```python
from build123d import *

# Parameters (mm, degrees)
SZKIC1_R                    = 23.5
DODANIE_WYCI_GNI_CIE1_DEPTH = 302
SZKIC2_R                    = 17.5
DODANIE_WYCI_GNI_CIE2_DEPTH = 50
SZKIC4_R                    = 17.5
DODANIE_WYCI_GNI_CIE3_DEPTH = 50
SZKIC5_R                    = 5.05
WYTNIJ_WYCI_GNI_CIE1_DEPTH  = 50
SFAZOWANIE1_SIZE            = 2
SZKIC8_R                    = 24
DODANIE_WYCI_GNI_CIE4_DEPTH = 42.129872
SZKIC12_R                   = 7
DODANIE_WYCI_GNI_CIE5_DEPTH = 61.69017
SZKIC6_R                    = 19
WYTNIJ_WYCI_GNI_CIE2_DEPTH  = 302
DODANIE_WYCI_GNI_CIE6_START = -50
SZKIC13_R                   = 7
DODANIE_WYCI_GNI_CIE6_DEPTH = 50


with BuildPart() as part:
    # Szkic1 → Dodanie-wyciągnięcie1 (new body)
    with BuildSketch(Plane(origin=(0, 0, 0), x_dir=(0, 0, -1), z_dir=(1, 0, 0))):
        Circle(SZKIC1_R)
    extrude(amount=DODANIE_WYCI_GNI_CIE1_DEPTH)

    # Szkic2 → Dodanie-wyciągnięcie2 (add)
    with BuildSketch(Plane.XY):
        with Locations(Location((31.5, -38, 0), (0, 0, 124.04773237))):
            Circle(SZKIC2_R)
    extrude(amount=DODANIE_WYCI_GNI_CIE2_DEPTH)

    # Szkic4 → Dodanie-wyciągnięcie3 (add)
    with BuildSketch(Plane(origin=(0, 0, 0), x_dir=(-1, 0, 0), z_dir=(0, 0, -1))):
        with Locations((-271.5, -38)):
            Circle(SZKIC4_R)
    extrude(amount=-DODANIE_WYCI_GNI_CIE3_DEPTH)

    # Szkic5 → Wytnij-wyciągnięcie1 (cut)
    with BuildSketch(Plane.XY.offset(50)):
        with Locations((31.5, -38)):
            Circle(SZKIC5_R)
        with Locations((271.5, -38)):
            Circle(SZKIC5_R)
    extrude(amount=-WYTNIJ_WYCI_GNI_CIE1_DEPTH, mode=Mode.SUBTRACT)

    # Sfazowanie1
    sfazowanie1_edges = [part.edges().sort_by_distance(p)[0] for p in [
        (26.45, -38, 0),
        (26.45, -38, 50),
        (266.45, -38, 0),
        (266.45, -38, 50),
    ]]
    chamfer(sfazowanie1_edges, length=SFAZOWANIE1_SIZE)

    # Szkic8 → Dodanie-wyciągnięcie4 (add)
    with BuildSketch(Plane(origin=(64.694528313, 23.5, 42), x_dir=(0.9969173337331281, 0, 0.07845909572784458), z_dir=(-0.07845909572784458, 0, 0.9969173337331281))):
        with Locations((0, -13.25)):
            Circle(SZKIC8_R)
    extrude(amount=-DODANIE_WYCI_GNI_CIE4_DEPTH)

    # Szkic12 → Dodanie-wyciągnięcie5 (add)
    with BuildSketch(Plane(origin=(-2.886875267, 0, 36.681228189), x_dir=(0.9969173337331281, 0, 0.07845909572784461), z_dir=(-0.07845909572784461, 0, 0.9969173337331281))):
        with Locations((67.790378694, 10.25)):
            Circle(SZKIC12_R)
    extrude(amount=DODANIE_WYCI_GNI_CIE5_DEPTH)

    # Szkic6 → Wytnij-wyciągnięcie2 (cut)
    with BuildSketch(Plane.ZY):
        Circle(SZKIC6_R)
    extrude(amount=-WYTNIJ_WYCI_GNI_CIE2_DEPTH, mode=Mode.SUBTRACT)

    # Szkic13 → Dodanie-wyciągnięcie6 (add)
    with BuildSketch(Plane(origin=(64.694528313, 23.5, 42), x_dir=(0.9969173337331281, 0, 0.07845909572784458), z_dir=(-0.07845909572784458, 0, 0.9969173337331281)).offset(DODANIE_WYCI_GNI_CIE6_START)):
        with Locations((0, -13.25)):
            Circle(SZKIC13_R)
    extrude(amount=DODANIE_WYCI_GNI_CIE6_DEPTH)


solid = part.part
```
Geometry check sheet. Reference: the model listing, model coordinates, mm. A direction names the side the tool comes from. Round coordinates to 2 decimals unless told otherwise and drop trailing zeros. Loops run counter-clockwise (first coordinate to the right, second up) from the corner with the lowest first, then second, coordinate; pieces in that order, holes last. Notation, with made-up numbers: (-12.5, -4.75) - (23.5, -4.75) arc R31 ccw to (23.5, 21.25) - close; hole circle Ø10 at (59, 51.5). An arc over 180 degrees is marked (long way). Write each question's results on one line, items separated by ' | '. Start each with the question number.
Q1. Release check for a two-part mould opening along Z. For faces 1 (the cylindrical face through (26.455, -37.778, 25.322)), 2 (the flat face through (272, -46, 0)), 3 (the conical face through (27.686, -34.502, 48.125)), 4 (the cylindrical face through (148.886, -16.856, 8.767)) record: +Z half, -Z half, draft (parallel to the pull), parting line (faces both ways), or undercut.
Q2. Cross-section at C-C on y = 0. Enter the section's corners in (x, z).
Q3. Gauge pin test, flat ends, axial feed: P1, Ø1, axis at x = 60.5, y = -16, coming from the -Z side; P2, Ø12, axis at x = 157, z = 23, coming from the +Y side (3 decimals); P3, Ø13, axis at x = 31.5, y = -38, coming from the +Z side; P4, Ø9, axis at x = 271.5, y = -38, coming from the +Z side. Record the tip position at first contact, or that the pin passes through.
Q4. Cross-section at A-A on y = -38. Enter the section's corners in (x, z), and give its area (3 significant figures).
Q5. Thickness scan on line 1 (Y direction, x = 271.5, z = 26); line 2 (Z direction, x = 170.5, y = 1.5); line 3 (Y direction, x = 282, z = 17.5). Record the ranges inside material, lowest first. Write a range as [from, to].
Q6. Cross-section at D-D on x = 123.5. Enter the section's corners in (y, z), and give its area (3 significant figures).
Q7. Access from +Z, -Z, +X, -X, +Y, -Y to the whole of each face (thin tool, end or side, straight path). Record for faces 5 (the cylindrical face through (148.89, -9, -21.71)), 6 (the flat face through (302, -17, -9)).
Q8. Cross-section at B-B on x = 31.5. Enter the section's corners in (y, z).
Answers below:
1) face 1: draft | face 2: -Z half | face 3: +Z half | face 4: undercut
2) outline: (0, -23.5) - (302, -23.5) - (302, -19) - (0, -19) - close; (0, 19) - (302, 19) - (302, 23.5) - (87.92, 23.5) - (86.33, 43.7) - (43.06, 40.3) - (44.38, 23.5) - (0, 23.5) - close
3) P1: stops at z = -17.66 | P2: stops at y = 16.225 | P3: stops at z = 49.45 | P4: passes through
4) outline: (14, 0) - (24.45, 0) - (26.45, 2) - (26.45, 48) - (24.45, 50) - (14, 50) - close; (36.55, 2) - (38.55, 0) - (49, 0) - (49, 50) - (38.55, 50) - (36.55, 48) - close; (254, 0) - (264.45, 0) - (266.45, 2) - (266.45, 48) - (264.45, 50) - (254, 50) - close; (276.55, 2) - (278.55, 0) - (289, 0) - (289, 50) - (278.55, 50) - (276.55, 48) - close | area: 2,470 mm²
5) line 1: y = [-55.5, -43.05], [-32.95, -20.5] | line 2: z = [-23.45, -18.94], [18.94, 23.45] | line 3: y = [-52, -24], [-15.68, -7.4], [7.4, 15.68]
6) outline: circle Ø47 at (0, 0); hole circle Ø38 at (0, 0) | area: 601 mm²
7) face 5: none | face 6: +Z, -Z, +X, +Y, -Y
8) outline: (-55.5, 0) - (-45.05, 0) - (-43.05, 2) - (-43.05, 48) - (-45.05, 50) - (-55.5, 50) - close; (-32.95, 2) - (-30.95, 0) - (-23.5, 0) arc R23.5 ccw (long way) to (-20.5, 11.49) - (-20.5, 50) - (-30.95, 50) - (-32.95, 48) - close; hole circle Ø38 at (0, 0)
